For this review, take the finished solid that the model builds, in its own axes (mm). Give positions to 0.01 mm unless a question says otherwise; leave off trailing zeros. Order: outer loops, then holes, each group sorted by start corner. A loop starts at its lowest first (then second) coordinate and runs counter-clockwise, first axis right, second up.
Item 1: For P1, Ø3.5, axis at x = 0, z = 584.2, coming from the +Y side; P2, Ø1.5, axis at x = -2.5, y = 2.5, coming from the +Z side, all flat-tipped, find the tip position at first contact; note any pin that passes through.
Item 2: Consider section A-A (z = 591). Give the boundary of the cut face in (x, y).
Item 3: For probe 1 along X at (y, z) = (-2.55, 584.2); probe 2 along X at (y, z) = (2, 409); probe 3 along Y at (x, z) = (-2.75, 548), list the stretches that pass through material, from the lowest coordinate up.
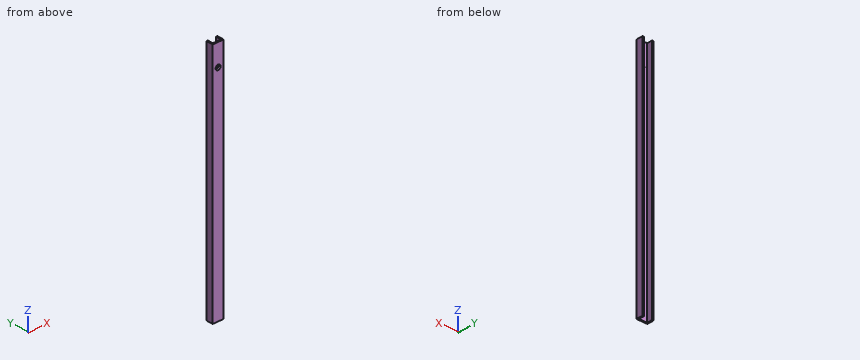
```python
from build123d import *

# Parameters (mm, degrees)
BOSS_EXTRUDE2_DEPTH = 609.6
SKETCH4_W           = 17.43115111
SKETCH4_H           = 13.311100502
CUT_EXTRUDE1_DEPTH  = 939.8
SKETCH5_R           = 1.5875
CUT_EXTRUDE2_DEPTH  = 610.684743459
CHAMFER1_SIZE       = 1.27


with BuildPart() as part:
    # Sketch3 → Boss-Extrude2 (new, symmetric)
    with BuildSketch(Plane.XY):
        Polygon((-6.35, 3.96875), (-6.35, -3.96875), (6.35, -3.96875), (6.35, 3.96875), (4.7625, 3.96875), (4.7625, -2.38125), (-4.7625, -2.38125), (-4.7625, 3.96875), align=None)
    extrude(amount=BOSS_EXTRUDE2_DEPTH, both=True)

    # Sketch4 → Cut-Extrude1 (cut)
    with BuildSketch(Plane.XY.offset(-609.6)):
        Rectangle(SKETCH4_W, SKETCH4_H)
    extrude(amount=CUT_EXTRUDE1_DEPTH, mode=Mode.SUBTRACT)

    # Sketch5 → Cut-Extrude2 (cut, through all)
    with BuildSketch(Plane.XZ.offset(3.96875)):
        with Locations(Location((0, 584.2, 0), (0, 0, 270))):
            Circle(SKETCH5_R)
    extrude(amount=-CUT_EXTRUDE2_DEPTH, mode=Mode.SUBTRACT)

    # Chamfer1
    chamfer1_edges = [part.edges().sort_by_distance(p)[0] for p in [
        (0, -3.96875, 585.7875),
    ]]
    chamfer(chamfer1_edges, length=CHAMFER1_SIZE)


solid = part.part
```
Resolved:
1. P1: stops at y = -2.38
1. P2: passes through
2. outline: (-6.35, -3.97) - (6.35, -3.97) - (6.35, 3.97) - (4.76, 3.97) - (4.76, -2.38) - (-4.76, -2.38) - (-4.76, 3.97) - (-6.35, 3.97) - close
3. probe 1: x = -6.35 to -1.59, 1.59 to 6.35
3. probe 2: x = -6.35 to -4.76, 4.76 to 6.35
3. probe 3: y = -3.97 to -2.38
